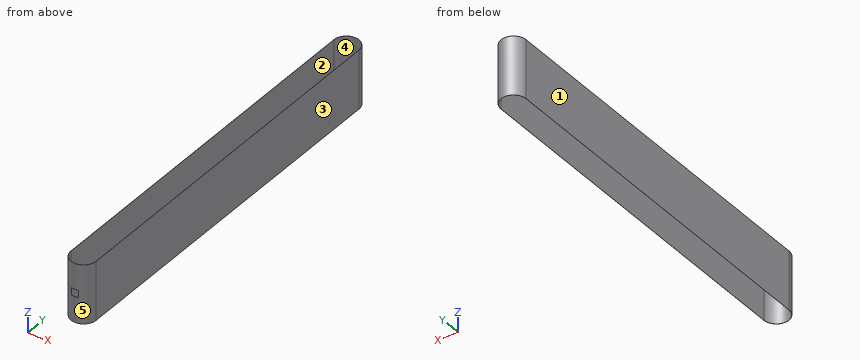
```python
from build123d import *

# Parameters (mm, degrees)
BOSS_EXTRUDE1_DEPTH = 40
SKETCH3_W           = 10
SKETCH3_H           = 10
CUT_EXTRUDE1_DEPTH  = 5


with BuildPart() as part:
    # Sketch1 → Boss-Extrude1 (new, symmetric)
    with BuildSketch(Plane.XY):
        with BuildLine():
            Line((-17.2, -250), (-17.2, 250))
            ThreePointArc((-17.2, 250), (0, 267.2), (17.2, 250))
            Line((17.2, 250), (17.2, -250))
            ThreePointArc((17.2, -250), (0, -267.2), (-17.2, -250))
        make_face()
        with BuildLine():
            Line((-17, -250), (-17, 250))
            ThreePointArc((-17, 250), (0, 267), (17, 250))
            Line((17, 250), (17, -250))
            ThreePointArc((17, -250), (0, -267), (-17, -250))
        make_face(mode=Mode.SUBTRACT)
    extrude(amount=BOSS_EXTRUDE1_DEPTH, both=True)

    # Sketch3 → Cut-Extrude1 (cut, symmetric)
    with BuildSketch(Plane.XY):
        with Locations((0, -267)):
            Rectangle(SKETCH3_W, SKETCH3_H)
    extrude(amount=CUT_EXTRUDE1_DEPTH, both=True, mode=Mode.SUBTRACT)


solid = part.part
```
Can you work these out from the model? Positions are in its coordinate system, mm. Face numbers are marked on the shaded views. A direction names the side the tool comes from. Coordinates: 2 decimals unless noted, no trailing zeros. Loops run counter-clockwise (first coordinate to the right, second up) from the corner with the lowest first, then second, coordinate; pieces in that order, holes last.
1) Imagine slicing it at B-B on x = 0. List the corners of the cut face in (y, z) for me.
2) Thinking about a two-plate mould opening in Y: for the marked faces 3, 4 and 5, which applies, pulls with the +Y half, pulls with the -Y half, needs draft (parallel to the pull), parting line crosses it, or undercut?
3) Imagine slicing it at C-C on z = 35. List the corners of the cut face in (x, y) for me.
4) I need wall thicknesses on probe 1 along X at (y, z) = (-132, -22); probe 2 along Y at (x, z) = (0.5, -16.5); probe 3 along Y at (x, z) = (2, 24). Which ranges of each line are inside material? Lowest first, please.
5) Which directions (+Z, -Z, +X, -X, +Y, -Y) give clear straight access to the entire face, cutting with the end or side of a thin tool? Please do the marked faces 1 and 2.
6) Imagine slicing it at A-A on y = -176. List the corners of the cut face in (x, z) for me.
7) For pin 1 (12 mm diameter, centred on x = -13, z = -7.5, fed in from -Y); pin 2 (0.5 mm diameter, centred on x = 0.5, y = -266.5, fed in from +Z); pin 3 (12 mm diameter, centred on x = -7.5, z = 12, fed in from +Y), each with a flat end and sliding along its axis, tell me the tip position at first contact or that it passes through.
Completed:
1. outline: (-267.2, -40) - (-267, -40) - (-267, -5) - (-267.2, -5) - close; (-267.2, 5) - (-267, 5) - (-267, 40) - (-267.2, 40) - close; (267, -40) - (267.2, -40) - (267.2, 40) - (267, 40) - close
2. face 3: needs draft
2. face 4: undercut
2. face 5: pulls with the -Y half
3. outline: (-17.2, -250) arc R17.2 ccw to (17.2, -250) - (17.2, 250) arc R17.2 ccw to (-17.2, 250) - close; hole (-17, -250) arc R17 ccw to (17, -250) - (17, 250) arc R17 ccw to (-17, 250) - close
4. probe 1: x = -17.2 to -17, 17 to 17.2
4. probe 2: y = -267.19 to -266.99, 266.99 to 267.19
4. probe 3: y = -267.08 to -266.88, 266.88 to 267.08
5. face 1: +Z, -Z, -X, +Y, -Y
5. face 2: +Z, -Z
6. outline: (-17.2, -40) - (-17, -40) - (-17, 40) - (-17.2, 40) - close; (17, -40) - (17.2, -40) - (17.2, 40) - (17, 40) - close
7. pin 1: stops at y = -265.71
7. pin 2: passes through
7. pin 3: stops at y = 267.13
